Geometry check sheet. Reference: drawing and pictorial views, mm from the part's lowest x, y, z. A direction names the side the tool comes from. Give positions to 0.01 mm unless a question says otherwise; leave off trailing zeros. Write each loop counter-clockwise with the first axis right and the second up, starting at its lowest first coordinate (ties: lowest second). Pieces come first, ordered by that corner, then holes. Notation, with made-up numbers: M 41.25,-17 L 81.25,-17 A20 cw 81.25,-10 Z; hole C 50.5,53.5 d10. An arc over 180 degrees is marked long. One line per item, written item: value. Start each with the question number.
1. Tool access check on the marked faces 4 and 5. Record the directions out of +Z, -Z, +X, -X, +Y, -Y that give a thin tool (end or side, any length) a straight path to the whole face; none if there is none.
2. Cross-section at D-D on y = 9.25. Record the cut outline in (x, z).
3. Scan lines: line 1 (X direction, y = 4.75, z = 5.9); line 2 (Y direction, x = 2.75, z = 6.25); line 3 (X direction, y = 16.5, z = 6) (1 decimal). Record each from-to range of solid material in increasing order.
4. Gauge pin test, flat ends, axial feed: pin 1 (2 mm diameter, centred on x = 9, y = 17.5, fed in from +Z); pin 2 (6 mm diameter, centred on x = 11.5, z = 6, fed in from +Y); pin 3 (0.6 mm diameter, centred on x = 15.5, y = 8.5, fed in from +Z); pin 4 (2 mm diameter, centred on x = 15, y = 14, fed in from -Z) (1 decimal). Record the tip position at first contact, or that the pin passes through.
5. Cross-section at A-A on x = 8. Record the cut outline in (y, z).
6. Cross-section at C-C on z = 7.25. Record the cut outline in (x, y).
7. Cross-section at B-B on y = 14.25. Record the cut outline in (x, z).
8. Release check for a two-part mould opening along Z. For the marked faces 1, 2 and 3 record: pulls with the +Z half, pulls with the -Z half, needs draft (parallel to the pull), parting line crosses it, or undercut.
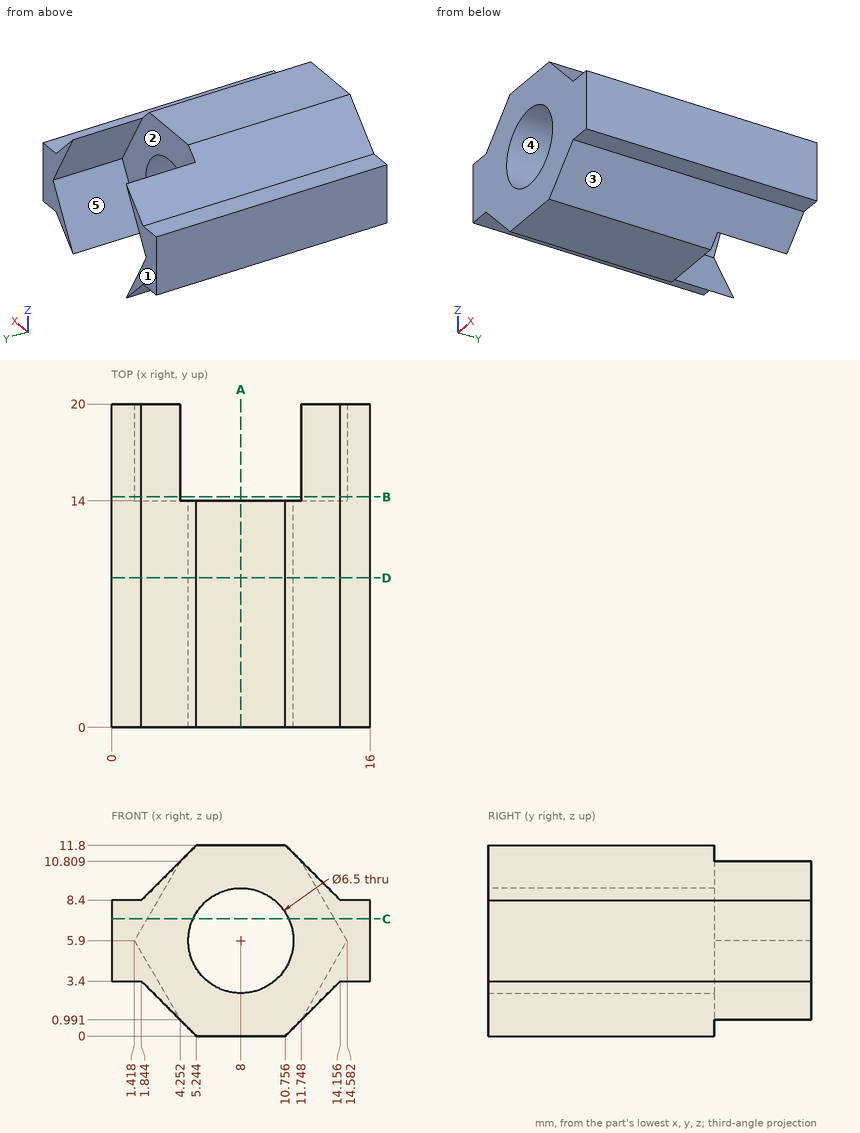
Report:
1. face 4: +Y, -Y
1. face 5: +Y
2. outline: M 0,3.4 L 1.84,3.4 L 5.24,0 L 10.76,0 L 14.16,3.4 L 16,3.4 L 16,8.4 L 14.16,8.4 L 10.76,11.8 L 5.24,11.8 L 1.84,8.4 L 0,8.4 Z; hole C 8,5.9 d6.5
3. line 1: x = 0 to 4.75, 11.25 to 16
3. line 2: y = 0 to 14
3. line 3: x = 0 to 1.5, 14.5 to 16
4. pin 1: passes through
4. pin 2: stops at y = 20
4. pin 3: stops at z = 8.4
4. pin 4: stops at z = 3.2
5. outline: M 0,0 L 14,0 L 14,2.65 L 0,2.65 Z; M 0,9.15 L 14,9.15 L 14,11.8 L 0,11.8 Z
6. outline: M 0,0 L 5.04,0 L 5.04,14 L 2.2,14 L 2.2,20 L 0,20 Z; M 10.96,0 L 16,0 L 16,20 L 13.8,20 L 13.8,14 L 10.96,14 Z
7. outline: M 0,3.4 L 1.84,3.4 L 4.25,0.99 L 1.42,5.9 L 4.25,10.81 L 1.84,8.4 L 0,8.4 Z; M 11.75,0.99 L 14.16,3.4 L 16,3.4 L 16,8.4 L 14.16,8.4 L 11.75,10.81 L 14.58,5.9 Z
8. face 1: needs draft
8. face 2: undercut
8. face 3: pulls with the -Z half
